Design review of the part built by this model. Coordinates are the model's own, in mm. Face numbers are marked on the shaded views. Round coordinates to 2 decimals unless told otherwise and drop trailing zeros. Loops run counter-clockwise (first coordinate to the right, second up) from the corner with the lowest first, then second, coordinate; pieces in that order, holes last. Notation, with made-up numbers: (-9.5, -2) - (7.5, -2) arc R34 ccw to (7.5, 33) - close; hole circle Ø3 at (19.25, 83). An arc over 180 degrees is marked (long way). Return JSON: item names as keys, results as strings. Group by question number.
(1) We need section D-D, the plane x = -25.5. Write out the cut boundary in (y, z).
(2) The part is to be moulded in two halves that separate along Z. For the marked faces 1, 2 and 3, say which applies: pulls with the +Z half, pulls with the -Z half, needs draft (parallel to the pull), parting line crosses it, or undercut.
(3) We need section A-A, the plane x = 0. Write out the cut boundary in (y, z), and give its area (3 significant figures).
(4) Clearance check with flat-ended pins moving along their axes: pin 1 (3 mm diameter, centred on y = 38.5, z = 5.5, fed in from -X); pin 2 (12 mm diameter, centred on x = -10.5, z = 3, fed in from +Y); pin 3 (8 mm diameter, centred on x = 14.5, z = 12, fed in from +Y); pin 4 (2 mm diameter, centred on x = 23.5, z = -10, fed in from -Y). State where each tip first meets the part, or that it passes through.
(5) Wall thickness on L1, parallel to Z at x = 0, y = 44; L2, parallel to Y at x = 3, z = 3.5: over which ranges is each line inside the solid? List them lowest first. Write a range as [from, to].
(6) We need section B-B, the plane z = 0. Write out the cut boundary in (x, y), and give its area (3 significant figures).
(7) We need section C-C, the plane y = 46. Write out the cut boundary in (x, z).
from build123d import *

# Parameters (mm, degrees)
BOSS_EXTRUDE1_DEPTH      = 31
BOSS_EXTRUDE1_DEPTH_BACK = 4
SKETCH7_R                = 10
SKETCH10_R               = 30
CUT_EXTRUDE1_DEPTH       = 47


# Read off the part's stored shape, not the designer's step: Shell1
with BuildPart() as part:
    # Sketch5 → Revolve3 (revolve)
    with BuildSketch(Plane(origin=(0, 0, 0), x_dir=(1, 0, 0), z_dir=(0, 1, 0))):
        with BuildLine():
            Line((0, -30), (0, 30))
            ThreePointArc((0, 30), (30, 0), (0, -30))
        make_face()
    revolve(axis=Axis((0, 0, 30), (0, 0, -1)))

    # Sketch7 → Boss-Extrude1 (add, two sides: drawn at the far end of the back side and taken through both)
    with BuildSketch(Plane(origin=(0, 30, 0), x_dir=(1, 0, 0), z_dir=(0, 1, 0)).offset(-BOSS_EXTRUDE1_DEPTH_BACK)):
        with Locations(Location((0, 0, 0), (0, 0, 270))):
            Circle(SKETCH7_R)
    extrude(amount=BOSS_EXTRUDE1_DEPTH + BOSS_EXTRUDE1_DEPTH_BACK)

    # Sketch10 → Cut-Extrude1 (cut)
    with BuildSketch(Plane(origin=(0, 0, 0), x_dir=(1, 0, 0), z_dir=(0, 1, 0))):
        Circle(SKETCH10_R)
    extrude(amount=-CUT_EXTRUDE1_DEPTH, mode=Mode.SUBTRACT)

    # Shell1 outline → Shell1 (revolve, cut)
    with BuildSketch(Plane.XY):
        with BuildLine():
            ThreePointArc((29, -2.9e-08), (23.473389189, 17.029386366), (8.999999972, 27.568097513))
            Line((8.999999972, 27.568097513), (9, 60))
            Line((9, 60), (0, 60))
            Line((0, 60), (0, -2.9e-08))
            Line((0, -2.9e-08), (29, -2.9e-08))
        make_face()
    revolve(axis=Axis((0, 0, 0), (0, 1, 0)), mode=Mode.SUBTRACT)


solid = part.part
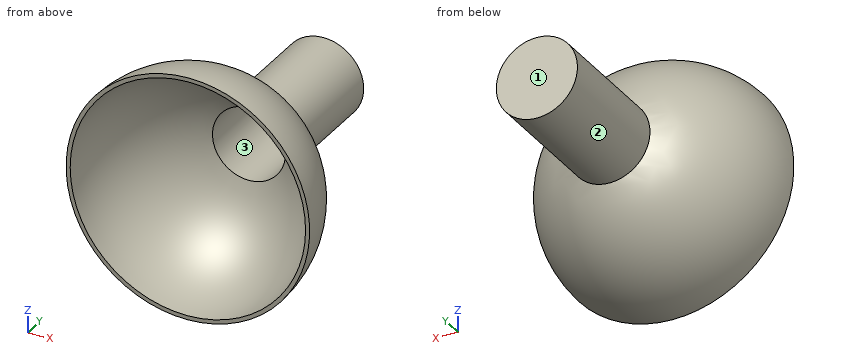
Solutions:
{
 "1": {"outline": "(0, -15.8) arc R15.8 ccw to (0, 15.8) - (0, 13.81) arc R13.81 cw to (0, -13.81) - close"},
 "2": {"face 1": "needs draft", "face 2": "parting line crosses it", "face 3": "undercut"},
 "3": {"outline": "(0, -30) arc R30 ccw to (28.28, -10) - (61, -10) - (61, 10) - (28.28, 10) arc R30 ccw to (0, 30) - (0, 29) arc R29 cw to (27.57, 9) - (60, 9) - (60, -9) - (27.57, -9) arc R29 cw to (0, -29) - close", "area": "157 mm^2"},
 "4": {"pin 1": "x = -9.17", "pin 2": "y = 61", "pin 3": "y = 26.08", "pin 4": "y = 11.69"},
 "5": {"L1": "[-10, -9], [9, 10]", "L2": "[60, 61]"},
 "6": {"outline": "(-30, 0) - (-29, 0) arc R29 cw to (-9, 27.57) - (-9, 60) - (9, 60) - (9, 27.57) arc R29 cw to (29, 0) - (30, 0) arc R30 ccw to (10, 28.28) - (10, 61) - (-10, 61) - (-10, 28.28) arc R30 ccw to start", "area": "157 mm^2"},
 "7": {"outline": "circle Ø20 at (0, 0); hole circle Ø18 at (0, 0)"}
}
